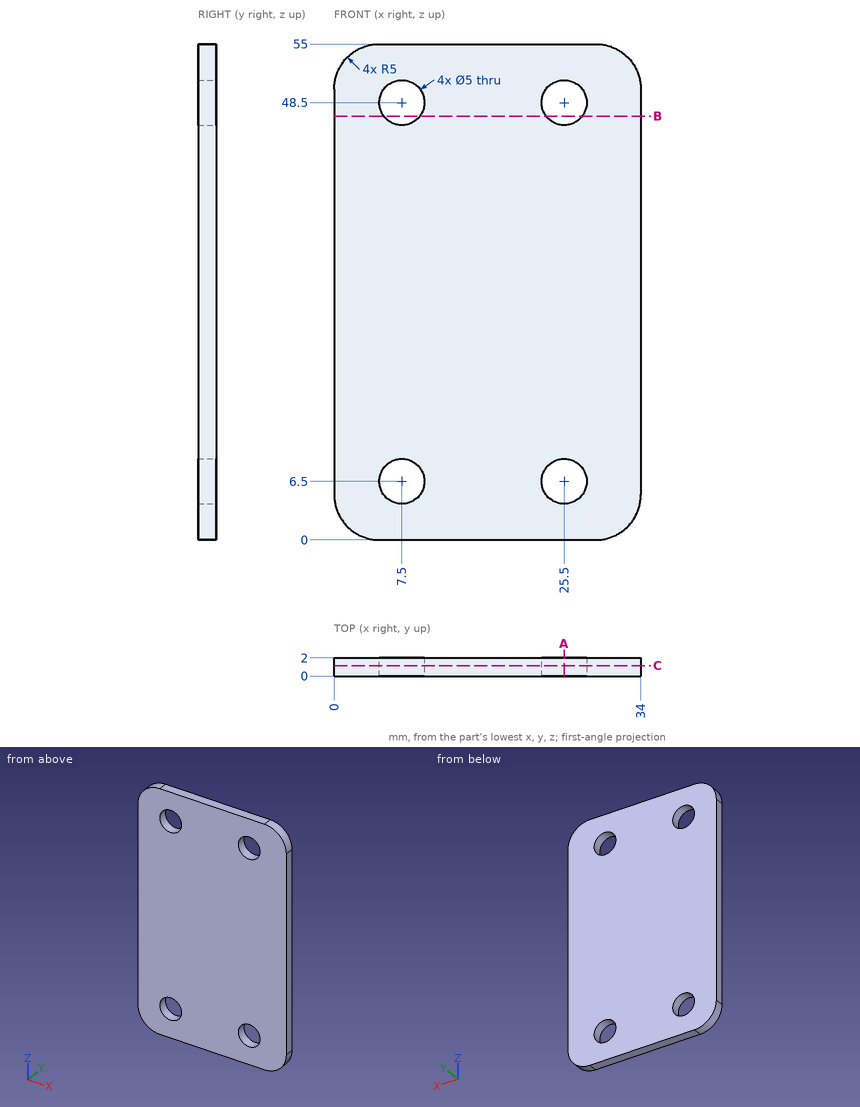
For this review, use the dimensioned drawing (mm, ordinates from the lowest corner) and the shaded views. Coordinates: 2 decimals unless noted, no trailing zeros. Order: outer loops, then holes, each group sorted by start corner. A loop starts at its lowest first (then second) coordinate and runs counter-clockwise, first axis right, second up. Notation, with made-up numbers: (83, 34.5) -> (114, 34.5) arc R15 cw to (114, 57.5) -> close; hole circle Ø7 at (49.25, 54). An arc over 180 degrees is marked (long way). One line per item, written item: value. Start each with the question number.
Q1. Take a section at B-B, the plane z = 47. State the section outline as (x, y) points, then the cut area to 3 significant figures.
Q2. Take a section at C-C, the plane y = 1.15. State the section outline as (x, z) points, then the cut area to 3 significant figures.
Q3. Take a section at A-A, the plane x = 25.5. State the section outline as (y, z) points, then the cut area to 3 significant figures.
Q4. For probe 1 along X at (y, z) = (0.55, 48.5); probe 2 along Z at (x, y) = (7.5, 0.65); probe 3 along Z at (x, y) = (7, 1.15), list the stretches that pass through material, from the lowest coordinate up.
Values follow:
1. outline: (0, 0) -> (5.5, 0) -> (5.5, 2) -> (0, 2) -> close; (9.5, 0) -> (23.5, 0) -> (23.5, 2) -> (9.5, 2) -> close; (27.5, 0) -> (34, 0) -> (34, 2) -> (27.5, 2) -> close
1. area: 52.0 mm2
2. outline: (0, 5) arc R5 ccw to (5, 0) -> (29, 0) arc R5 ccw to (34, 5) -> (34, 50) arc R5 ccw to (29, 55) -> (5, 55) arc R5 ccw to (0, 50) -> close; hole circle Ø5 at (7.5, 6.5); hole circle Ø5 at (7.5, 48.5); hole circle Ø5 at (25.5, 6.5); hole circle Ø5 at (25.5, 48.5)
2. area: 1,770 mm2
3. outline: (0, 0) -> (2, 0) -> (2, 4) -> (0, 4) -> close; (0, 9) -> (2, 9) -> (2, 46) -> (0, 46) -> close; (0, 51) -> (2, 51) -> (2, 55) -> (0, 55) -> close
3. area: 90.0 mm2
4. probe 1: x = 0 to 5, 10 to 23, 28 to 34
4. probe 2: z = 0 to 4, 9 to 46, 51 to 55
4. probe 3: z = 0 to 4.05, 8.95 to 46.05, 50.95 to 55
